Part print with two shaded views. Sizes in mm from the minimum x, y, z corner. A direction names the side the tool comes from. Give positions to 0.01 mm unless a question says otherwise; leave off trailing zeros. Loops run counter-clockwise (first coordinate to the right, second up) from the corner with the lowest first, then second, coordinate; pieces in that order, holes last. Notation, with made-up numbers: M 4.25,-5.75 L 27.25,-5.75 A26 cw 27.25,22.25 Z; hole C 37.25,1.25 d11. An arc over 180 degrees is marked long. Answer in a Markdown table with one row per item.
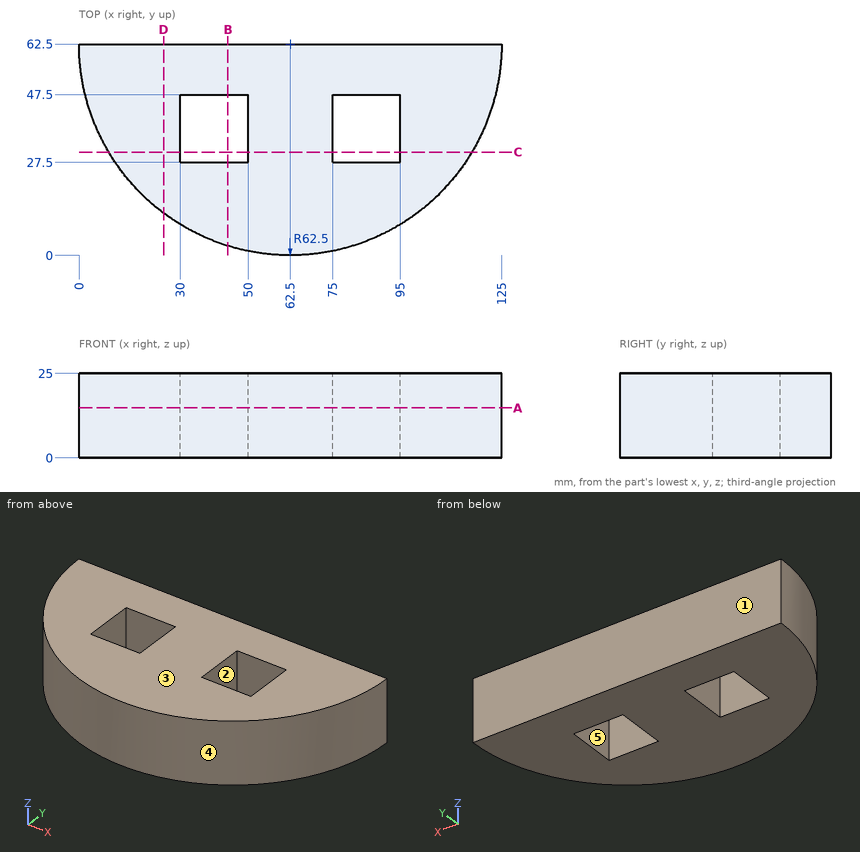
Q1. Saw through at B-B (x = 44). Give the cut face in (y, z), and give its area (3 significant figures).
Reported:
| item | result |
|---|---|
| outline | M 2.8,0 L 27.5,0 L 27.5,25 L 2.8,25 Z; M 47.5,0 L 62.5,0 L 62.5,25 L 47.5,25 Z |
| area | 992 mm² |
Q2. Mould opens along X. For the marked faces 3, 4 and 5 say: released by +X, released by -X, zero draft, split by the parting line, or undercut.
Reported:
| item | result |
|---|---|
| face 3 | zero draft |
| face 4 | split by the parting line |
| face 5 | undercut |
Q3. Saw through at C-C (y = 30.5). Give the cut face in (x, z), and give its area (3 significant figures).
Reported:
| item | result |
|---|---|
| outline | M 8.81,0 L 30,0 L 30,25 L 8.81,25 Z; M 50,0 L 75,0 L 75,25 L 50,25 Z; M 95,0 L 116.19,0 L 116.19,25 L 95,25 Z |
| area | 1,680 mm² |
Q4. Drop flat-ended pins along their axis: pin 1 (10 mm diameter, centred on y = 41, z = 18, fed in from +X); pin 2 (2 mm diameter, centred on y = 43.5, z = 8, fed in from -X); pin 3 (6 mm diameter, centred on x = 35.5, z = 17, fed in from -Y). Give the stop position or say it passes through.
Reported:
| item | result |
|---|---|
| pin 1 | x = 122.78 |
| pin 2 | x = 2.65 |
| pin 3 | y = 4.79 |
Q5. Probe probe 1 along X at (y, z) = (42, 8.5); probe 2 along X at (y, z) = (35, 2.75); probe 3 along Y at (x, z) = (37, 19.5). List the from-to ranges inside material, lowest first.
Reported:
| item | result |
|---|---|
| probe 1 | 3.46 to 30, 50 to 75, 95 to 121.54 |
| probe 2 | 6.38 to 30, 50 to 75, 95 to 118.62 |
| probe 3 | 5.44 to 27.5, 47.5 to 62.5 |
Q6. 3-axis set-ups, long thin cutter, end or side, ignore diameter. For the marked faces 1 and 2: which of +Z, -Z, +X, -X, +Y, -Y reach the whole face in a straight line?
Reported:
| item | result |
|---|---|
| face 1 | +Z, -Z, +X, -X, +Y |
| face 2 | +Z, -Z |
Q7. Saw through at D-D (x = 25). Give the cut face in (y, z), and give its area (3 significant figures).
Reported:
| item | result |
|---|---|
| outline | M 12.5,0 L 62.5,0 L 62.5,25 L 12.5,25 Z |
| area | 1,250 mm² |
Q8. Saw through at A-A (z = 14.75). Give the cut face in (x, y).
Reported:
| item | result |
|---|---|
| outline | M 0,62.5 A62.5 ccw 125,62.5 Z; hole M 30,27.5 L 50,27.5 L 50,47.5 L 30,47.5 Z; hole M 75,27.5 L 95,27.5 L 95,47.5 L 75,47.5 Z |
